```python
from build123d import *

# Parameters (mm, degrees)
PAD037_DEPTH    = 65
PAD038_DEPTH    = 13
SKETCH098_R     = 4
POCKET036_DEPTH = 32.5
SKETCH099_R     = 3.15
POCKET037_DEPTH = 75
POCKET038_DEPTH = 65
PAD040_DEPTH    = 18
POCKET039_DEPTH = 6


with BuildPart() as part:
    # Sketch095 → Pad037 (new body)
    with BuildSketch(Plane.XZ.offset(66)):
        with BuildLine():
            Line((8, 17.868052), (-3.5, 17.868052))
            ThreePointArc((-3.5, 17.868052), (-4.914214, 17.282266), (-5.5, 15.868052))
            Line((-5.5, 15.868052), (-5.5, -6))
            ThreePointArc((-5.5, -6), (-4.914214, -7.414214), (-3.5, -8))
            Line((-3.5, -8), (8, -8))
            ThreePointArc((8, -8), (9.414214, -7.414214), (10, -6))
            Line((10, -6), (10, 15.868052))
            ThreePointArc((10, 15.868052), (9.414214, 17.282266), (8, 17.868052))
        make_face()
    extrude(amount=-PAD037_DEPTH)

    # Sketch096 → Pad038 (join)
    with BuildSketch(Plane.XY.offset(1)):
        Polygon((-4.849713, -30.253677), (-4.849713, -1.120098), (-13.449671, -30.253677), align=None)
    extrude(amount=PAD038_DEPTH)

    # Sketch098 → Pocket036 (cut, symmetric)
    with BuildSketch(Plane(origin=(0, -37, 7.42), x_dir=(0, 1, 0), z_dir=(1, 0, 0))):
        Circle(SKETCH098_R)
    extrude(amount=POCKET036_DEPTH, both=True, mode=Mode.SUBTRACT)

    # Sketch099 → Pocket037 (cut)
    with BuildSketch(Plane.XZ.offset(1)):
        Circle(SKETCH099_R)
    extrude(amount=POCKET037_DEPTH, mode=Mode.SUBTRACT)

    # Sketch100 → Pocket038 (cut)
    with BuildSketch(Plane.XZ.offset(1)):
        Polygon((-6.320894, 20), (1.017517, 20), (1.017517, 0), (0.034595, 0), (0.034595, 16.403641), (-6.320894, 16.403641), align=None)
    extrude(amount=POCKET038_DEPTH, mode=Mode.SUBTRACT)

    # Sketch103 → Pad040 (join)
    with BuildSketch(Plane.XY.offset(-8)):
        with BuildLine():
            Line((6.490593, -32.616061), (6.490593, -66))
            Line((6.490593, -66), (18.841947, -66))
            ThreePointArc((18.841947, -66), (28.302274, -62.640542), (33.525058, -54.066961))
            Line((33.525058, -54.066961), (39.008216, -27.816282))
            ThreePointArc((39.008216, -27.816282), (35.177971, -21.90851), (29.23767, -25.688111))
            Line((29.23767, -25.688111), (24.814264, -45.192815))
            ThreePointArc((10, -43.534037), (16.665428, -50.987459), (24.814264, -45.192815))
            Line((10, -43.534037), (10, -32.616061))
            Line((6.490593, -32.616061), (10, -32.616061))
        make_face()
    extrude(amount=PAD040_DEPTH)

    # Sketch102 → Pocket039 (cut)
    with BuildSketch(Plane(origin=(10, -37, 7.42), x_dir=(0, 1, 0), z_dir=(1, 0, 0))):
        Polygon((0, 7.621024), (-6.6, 3.810512), (-6.6, -3.810512), (0, -7.621024), (6.6, -3.810512), (6.6, 3.810512), align=None)
    extrude(amount=-POCKET039_DEPTH, mode=Mode.SUBTRACT)


with BuildPart() as part_1:
    # Body022 placement: moved
    add(part.part.moved(Location((33, 20, -24))))


solid = part_1.part
```
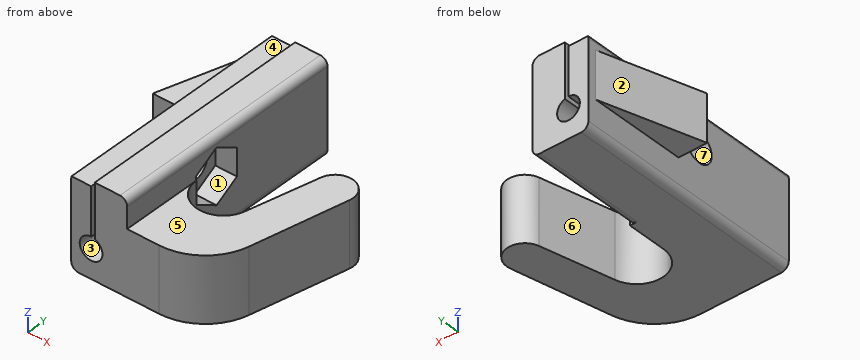
Here's how the part is built. I have some questions about the finished solid (model axes, mm). Face numbers are marked on the shaded views. A direction names the side the tool comes from. Round coordinates to 2 decimals unless told otherwise and drop trailing zeros. Order: outer loops, then holes, each group sorted by start corner. A loop starts at its lowest first (then second) coordinate and runs counter-clockwise, first axis right, second up. Notation, with made-up numbers: (15, 1) -> (36, 1) arc R31 cw to (36, 26) -> close; hole circle Ø7 at (18, 38). An arc over 180 degrees is marked (long way). Use a Markdown table: item, result. Add a question column.
(1) Suppose I cut it at B-B, the plane y = -30. Please give me the cut outline in (x, z).
(2) If we mould it in two halves opening along Z, with no side actions, what happens to the marked faces 1, 2, 3 and 4? For each: released by +Z, released by -Z, zero draft, split by the parting line, or undercut.
(3) I need wall thicknesses on line 1 along Z through (x, y) = (31.85, -17); line 2 along Z through (x, y) = (29.8, -17); line 3 along X through (y, z) = (-24.5, -24). Which ranges of each line are inside material? Lowest first, please.
(4) Suppose I cut it at A-A, the plane z = -16.58. Please give me the cut outline in (x, y).
(5) For pin 1 Ø14.5 at (y, z) = (-25, -17) entering from +X; pin 2 Ø9 at (y, z) = (-17, -16.58) entering from +X; pin 3 Ø12 at (x, y) = (64.5, -23.5) entering from +Z, each with a flat end and sliding along its axis, tell me the tip position at first contact or that it passes through.
(6) Suppose I cut it at D-D, the plane y = 0. Please give me the cut outline in (x, z).
(7) For the marked faces 5, 6 and 7, which set-ups out of +Z, -Z, +X, -X, +Y, -Y let a thin tool reach every point of the face, with its end or its side?
(8) Suppose I cut it at C-C, the plane z = -28.5. Please give me the cut outline in (x, y), and give its area (3 significant figures).
Verdict:
| question | item | result |
|---|---|---|
| 1 | outline | (27.5, -30) arc R2 ccw to (29.5, -32) -> (46.7, -32) -> (46.7, -14) -> (43, -14) -> (43, -8.13) arc R2 ccw to (41, -6.13) -> (34.02, -6.13) -> (34.02, -21.02) arc R3.15 cw (long way) to (33.03, -20.85) -> (33.03, -7.6) -> (27.57, -7.6) arc R2 ccw to (27.5, -8.13) -> close; (54.3, -32) -> (67.37, -32) -> (67.37, -14) -> (54.3, -14) -> close |
| 2 | face 1 | undercut |
| 2 | face 2 | zero draft |
| 2 | face 3 | undercut |
| 2 | face 4 | released by +Z |
| 3 | line 1 | -32 to -26.93, -21.07 to -20.58, -12.58 to -7.6 |
| 3 | line 2 | -32 to -20.58, -12.58 to -7.6 |
| 3 | line 3 | 27.5 to 29.85, 36.15 to 43.06, 57.97 to 68.52 |
| 4 | outline | (19.55, -10.25) -> (27.5, -10.25) -> (27.5, -13) -> (33.03, -13) -> (33.03, 19) -> (27.5, 19) -> (27.5, 16.68) -> close; (27.5, -46) -> (33.03, -46) -> (33.03, -21) -> (27.5, -21) -> close; (34.02, -46) -> (51.84, -46) arc R15 ccw to (66.53, -34.07) -> (72.01, -7.82) arc R5 ccw to (62.24, -5.69) -> (57.81, -25.19) arc R7.5 cw to (43, -23.53) -> (43, -23.6) -> (37, -23.6) -> (37, -21) -> (34.02, -21) -> close; (34.02, -13) -> (37, -13) -> (37, -10.4) -> (43, -10.4) -> (43, 19) -> (34.02, 19) -> close |
| 5 | pin 1 | x = 69.93 |
| 5 | pin 2 | x = 71.03 |
| 5 | pin 3 | z = -14 |
| 6 | outline | (22.58, -23) -> (27.5, -23) -> (27.5, -30) arc R2 ccw to (29.5, -32) -> (41, -32) arc R2 ccw to (43, -30) -> (43, -8.13) arc R2 ccw to (41, -6.13) -> (34.02, -6.13) -> (34.02, -21.02) arc R3.15 cw (long way) to (33.03, -20.85) -> (33.03, -7.6) -> (27.57, -7.6) arc R2 ccw to (27.5, -8.13) -> (27.5, -10) -> (22.58, -10) -> close |
| 7 | face 5 | +Z, +X, +Y, -Y |
| 7 | face 6 | +Z, -Z, +Y |
| 7 | face 7 | -X |
| 8 | outline | (27.5, -46) -> (51.84, -46) arc R15 ccw to (66.53, -34.07) -> (72.01, -7.82) arc R5 ccw to (62.24, -5.69) -> (57.81, -25.19) arc R7.5 cw to (43, -23.53) -> (43, 19) -> (27.5, 19) -> close |
| 8 | area | 1,630 mm2 |
